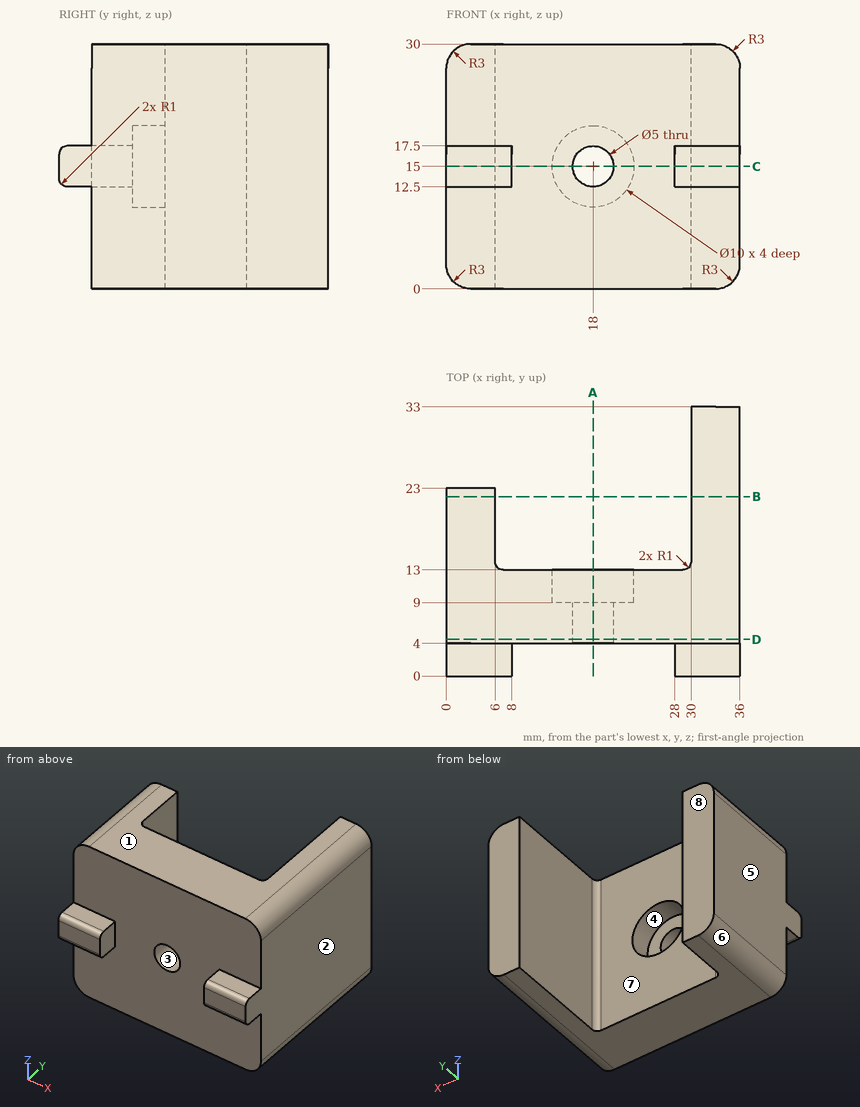
Verification items for this drawing (mm, ordinates from the low corner). A direction names the side the tool comes from. Round coordinates to 2 decimals unless told otherwise and drop trailing zeros. Order: outer loops, then holes, each group sorted by start corner. A loop starts at its lowest first (then second) coordinate and runs counter-clockwise, first axis right, second up. Notation, with made-up numbers: (21.25, 9) - (52.25, 9) arc R32 ccw to (52.25, 43) - close; hole circle Ø3 at (-11, 36). An arc over 180 degrees is marked (long way). Answer as CSV lines item,"result". Start each with the question number.
1) Section check A-A (x = 18). Record the cut outline in (y, z), then the cut area to 3 significant figures.
2) Draft check along X on the marked faces 1, 2 and 3. Enter one of: +X half, -X half, draft (parallel to the pull), parting line (faces both ways), or undercut.
3) Depth check by flat-ended pin: pin 1 (8 mm diameter, centred on x = 18, z = 12, fed in from -Y); pin 2 (8 mm diameter, centred on x = 20, z = 13, fed in from +Y); pin 3 (2.5 mm diameter, centred on x = 4, y = 2.5, fed in from +Z); pin 4 (4 mm diameter, centred on x = 25.5, y = 16, fed in from +Z). Enter the tip coordinate at first touch or a pass-through.
4) Tool access check on the marked faces 4, 5, 6, 7 and 8. Record the directions out of +Z, -Z, +X, -X, +Y, -Y that give a thin tool (end or side, any length) a straight path to the whole face; none if there is none.
5) Section check C-C (z = 15). Record the cut outline in (x, y).
6) Section check B-B (y = 22). Record the cut outline in (x, z).
7) Section check D-D (y = 4.5). Record the cut outline in (x, z).
8) Scan lines: probe 1 along X at (y, z) = (21, 19.75); probe 2 along X at (y, z) = (11.95, 15); probe 3 along Y at (x, z) = (10, 17.25). Record each from-to range of solid material in increasing order.
Determined:
1,outline,"(4, 0) - (13, 0) - (13, 10) - (9, 10) - (9, 12.5) - (4, 12.5) - close; (4, 17.5) - (9, 17.5) - (9, 20) - (13, 20) - (13, 30) - (4, 30) - close"
1,area,"205 mm^2"
2,face 1,"draft"
2,face 2,"+X half"
2,face 3,"undercut"
3,pin 1,"y = 4"
3,pin 2,"y = 13"
3,pin 3,"z = 17.5"
3,pin 4,"through"
4,face 4,"+Y"
4,face 5,"+Z, -Z, -X, +Y, -Y"
4,face 6,"-Z, -X, +Y, -Y"
4,face 7,"+Z, -Z, +Y"
4,face 8,"+Z, -Z, -X, +Y"
5,outline,"(0, 0) - (8, 0) - (8, 4) - (15.5, 4) - (15.5, 9) - (13, 9) - (13, 13) - (7, 13) arc R1 cw to (6, 14) - (6, 23) - (0, 23) - close; (20.5, 4) - (28, 4) - (28, 0) - (36, 0) - (36, 33) - (30, 33) - (30, 14) arc R1 cw to (29, 13) - (23, 13) - (23, 9) - (20.5, 9) - close"
6,outline,"(0, 3) arc R3 ccw to (3, 0) - (6, 0) - (6, 30) - (3, 30) arc R3 ccw to (0, 27) - close; (30, 0) - (33, 0) arc R3 ccw to (36, 3) - (36, 27) arc R3 ccw to (33, 30) - (30, 30) - close"
7,outline,"(0, 3) arc R3 ccw to (3, 0) - (33, 0) arc R3 ccw to (36, 3) - (36, 27) arc R3 ccw to (33, 30) - (3, 30) arc R3 ccw to (0, 27) - close; hole circle Ø5 at (18, 15)"
8,probe 1,"0 to 6, 30 to 36"
8,probe 2,"0 to 13, 23 to 36"
8,probe 3,"4 to 13"
